Here's how the part is built. I have some questions about the finished solid (model axes, mm). Face numbers are marked on the shaded views. A direction names the side the tool comes from. Round coordinates to 2 decimals unless told otherwise and drop trailing zeros. Loops run counter-clockwise (first coordinate to the right, second up) from the corner with the lowest first, then second, coordinate; pieces in that order, holes last. Notation, with made-up numbers: (-27.75, 43.25) - (10.25, 43.25) arc R27 cw to (10.25, 73.25) - close; hole circle Ø4 at (48, -11). An arc over 180 degrees is marked (long way). Return JSON: item names as keys, results as strings. Group by question number.
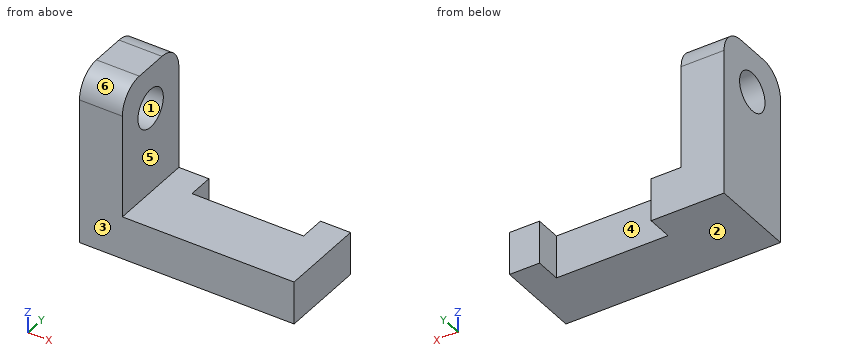
```python
from build123d import *

# Parameters (mm, degrees)
F1_DEPTH = 5
F2_W     = 5
F2_H     = 10
F3_DEPTH = 15
F4_R     = 2.25
F5_DEPTH = 25
F6_R     = 3


with BuildPart() as f1:
    # F0 (on Top) → F1 (new body)
    with BuildSketch(Plane.XY):
        Polygon((-15.6191263039, -2.0692273974), (-15.6191263039, -12.0692273974), (9.3808736961, -12.0692273974), (9.3808736961, -2.0692273974), (5.8808736961, -2.0692273974), (5.8808736961, -5.0692273974), (-7.1191263039, -5.0692273974), (-7.1191263039, -2.0692273974), align=None)
    extrude(amount=F1_DEPTH)

    # F2 (on face) → F3 (join)
    with BuildSketch(Plane.XY.offset(5)):
        with Locations((-13.1191263039, -7.0692273974)):
            Rectangle(F2_W, F2_H)
    extrude(amount=F3_DEPTH)

    # F4 (on face) → F5 (cut)
    with BuildSketch(Plane(origin=(-15.6191263039, 0, 0), x_dir=(0, -1, 0), z_dir=(-1, 0, 0))):
        with Locations((7.0692273974, 15)):
            Circle(F4_R)
    extrude(amount=-F5_DEPTH, mode=Mode.SUBTRACT)

    # F6
    f6_edges = [f1.edges().sort_by_distance(p)[0] for p in [
        (-13.119126, -12.069227, 20),
        (-13.119126, -2.069227, 20),
    ]]
    fillet(f6_edges, radius=F6_R)


solid = f1.part
```
Q1. For the marked faces 4, 5 and 6, which set-ups out of +Z, -Z, +X, -X, +Y, -Y let a thin tool reach every point of the face, with its end or its side?
Q2. Imagine slicing it at D-D, the plane x = 5.25. List the corners of the cut face in (y, z) for me, and give its area (3 significant figures).
Q3. Will these pins go through, and if not, where does the flat tip stop? pin 1 Ø3 at (x, y) = (3, -7.5) entering from -Z; pin 2 Ø4 at (x, y) = (-2, -10) entering from +Z; pin 3 Ø6 at (y, z) = (-7.07, 15) entering from +X; pin 4 Ø1.5 at (x, z) = (-1.5, 1.5) entering from +Y.
Q4. Imagine slicing it at A-A, the plane y = -7. List the corners of the cut face in (x, z) for me.
Q5. Imagine slicing it at B-B, the plane z = 15. List the corners of the cut face in (x, y) for me, and give its area (3 significant figures).
Q6. Imagine slicing it at C-C, the plane x = -13.25. List the corners of the cut face in (y, z) for me, and give its area (3 significant figures).
Q7. If we mould it in two halves opening along Y, with no side actions, what happens to the marked faces 1, 2 and 3? For each: +Y half, -Y half, draft (parallel to the pull), parting line (faces both ways), or undercut.
Q8. Please list where these lines run through material, in increasing order: line 1 (X direction, y = -4.5, z = 3.5); line 2 (X direction, y = -8.25, z = 12.5); line 3 (Z direction, x = -3, y = -6.75).
Output values:
{
 "1": {"face 4": "+Z, -Z, +Y", "face 5": "+Z, +X, +Y, -Y", "face 6": "+Z, +X, -X, -Y"},
 "2": {"outline": "(-12.07, 0) - (-5.07, 0) - (-5.07, 5) - (-12.07, 5) - close", "area": "35.0 mm^2"},
 "3": {"pin 1": "stops at z = 0", "pin 2": "stops at z = 5", "pin 3": "stops at x = -10.62", "pin 4": "stops at y = -5.07"},
 "4": {"outline": "(-15.62, 0) - (9.38, 0) - (9.38, 5) - (-10.62, 5) - (-10.62, 12.75) - (-15.62, 12.75) - close; (-15.62, 17.25) - (-10.62, 17.25) - (-10.62, 20) - (-15.62, 20) - close"},
 "5": {"outline": "(-15.62, -12.07) - (-10.62, -12.07) - (-10.62, -9.32) - (-15.62, -9.32) - close; (-15.62, -4.82) - (-10.62, -4.82) - (-10.62, -2.07) - (-15.62, -2.07) - close", "area": "27.5 mm^2"},
 "6": {"outline": "(-12.07, 0) - (-2.07, 0) - (-2.07, 17) arc R3 ccw to (-5.07, 20) - (-9.07, 20) arc R3 ccw to (-12.07, 17) - close; hole circle Ø4.5 at (-7.07, 15)", "area": "180 mm^2"},
 "7": {"face 1": "undercut", "face 2": "draft", "face 3": "-Y half"},
 "8": {"line 1": "x = -15.62 to -7.12, 5.88 to 9.38", "line 2": "x = -15.62 to -10.62", "line 3": "z = 0 to 5"}
}
